```python
from build123d import *

# Parameters (mm, degrees)
SKETCH1_W                      = 560
SKETCH1_H                      = 450
BOSS_EXTRUDE1_DEPTH            = 20
SKETCH3_W                      = 20
SKETCH3_H                      = 450
BOSS_EXTRUDE2_DEPTH            = 120
LPATTERN2_COUNT                = 7
LPATTERN2_PITCH                = 140
LPATTERN5_COUNT                = 2
LPATTERN5_PITCH                = 270
LPATTERN5_COUNT_DIR2           = 14
LPATTERN5_PITCH_DIR2           = 140
SKETCH6_W                      = 450
SKETCH6_H                      = 1000
BOSS_EXTRUDE5_DEPTH            = 20
BOSS_EXTRUDE6_DEPTH            = 450
CUT_EXTRUDE1_REACH             = 1486.158
SKETCH10_R                     = 4.4
CUT_EXTRUDE1_DIRECTION_2_REACH = 1486.158
LPATTERN6_COUNT                = 3
LPATTERN6_PITCH                = 270
SKETCH13_W                     = 315
SKETCH13_H                     = 1.2
CUT_EXTRUDE3_DEPTH             = 20


with BuildPart() as part:
    # Sketch1 → Boss-Extrude1 (new body)
    with BuildSketch(Plane(origin=(0, 0, 0), x_dir=(1, 0, 0), z_dir=(0, 1, 0))):
        Rectangle(SKETCH1_W, SKETCH1_H)
    boss_extrude1 = extrude(amount=BOSS_EXTRUDE1_DEPTH)

    # Sketch3 → Boss-Extrude2 (add)
    with BuildSketch(Plane(origin=(0, 20, 0), x_dir=(1, 0, 0), z_dir=(0, 1, 0))):
        with Locations((-270, 0)):
            Rectangle(SKETCH3_W, SKETCH3_H)
        Rectangle(SKETCH3_W, SKETCH3_H)
        with Locations((270, 0)):
            Rectangle(SKETCH3_W, SKETCH3_H)
    extrude(amount=BOSS_EXTRUDE2_DEPTH)


with BuildPart() as lpattern2_1:
    # LPattern2: pattern copy
    add(part.part.moved(Location(Vector(0, 1, 0) * (1 * LPATTERN2_PITCH))))


with BuildPart() as lpattern2_2:
    # LPattern2: pattern copy
    add(part.part.moved(Location(Vector(0, 1, 0) * (2 * LPATTERN2_PITCH))))


with BuildPart() as lpattern2_3:
    # LPattern2: pattern copy
    add(part.part.moved(Location(Vector(0, 1, 0) * (3 * LPATTERN2_PITCH))))


with BuildPart() as lpattern2_4:
    # LPattern2: pattern copy
    add(part.part.moved(Location(Vector(0, 1, 0) * (4 * LPATTERN2_PITCH))))


with BuildPart() as lpattern2_5:
    # LPattern2: pattern copy
    add(part.part.moved(Location(Vector(0, 1, 0) * (5 * LPATTERN2_PITCH))))


with BuildPart() as lpattern2_6:
    # LPattern2: pattern copy
    add(part.part.moved(Location(Vector(0, 1, 0) * (6 * LPATTERN2_PITCH))))


with BuildPart() as lpattern5_1:
    # LPattern5: pattern copy
    add(boss_extrude1.moved(Location(Vector(1, 0, 0) * (0 * LPATTERN5_PITCH) + Vector(0, 1, 0) * (1 * LPATTERN5_PITCH_DIR2))))


with BuildPart() as lpattern5_2:
    # LPattern5: pattern copy
    add(boss_extrude1.moved(Location(Vector(1, 0, 0) * (0 * LPATTERN5_PITCH) + Vector(0, 1, 0) * (2 * LPATTERN5_PITCH_DIR2))))


with BuildPart() as lpattern5_3:
    # LPattern5: pattern copy
    add(boss_extrude1.moved(Location(Vector(1, 0, 0) * (0 * LPATTERN5_PITCH) + Vector(0, 1, 0) * (3 * LPATTERN5_PITCH_DIR2))))


with BuildPart() as lpattern5_4:
    # LPattern5: pattern copy
    add(boss_extrude1.moved(Location(Vector(1, 0, 0) * (0 * LPATTERN5_PITCH) + Vector(0, 1, 0) * (4 * LPATTERN5_PITCH_DIR2))))


with BuildPart() as lpattern5_5:
    # LPattern5: pattern copy
    add(boss_extrude1.moved(Location(Vector(1, 0, 0) * (0 * LPATTERN5_PITCH) + Vector(0, 1, 0) * (5 * LPATTERN5_PITCH_DIR2))))


with BuildPart() as lpattern5_6:
    # LPattern5: pattern copy
    add(boss_extrude1.moved(Location(Vector(1, 0, 0) * (0 * LPATTERN5_PITCH) + Vector(0, 1, 0) * (6 * LPATTERN5_PITCH_DIR2))))


with BuildPart() as lpattern5_7:
    # LPattern5: pattern copy
    add(boss_extrude1.moved(Location(Vector(1, 0, 0) * (0 * LPATTERN5_PITCH) + Vector(0, 1, 0) * (7 * LPATTERN5_PITCH_DIR2))))


with BuildPart() as lpattern5_8:
    # LPattern5: pattern copy
    add(boss_extrude1.moved(Location(Vector(1, 0, 0) * (1 * LPATTERN5_PITCH) + Vector(0, 1, 0) * (0 * LPATTERN5_PITCH_DIR2))))


with BuildPart() as lpattern5_9:
    # LPattern5: pattern copy
    add(boss_extrude1.moved(Location(Vector(1, 0, 0) * (1 * LPATTERN5_PITCH) + Vector(0, 1, 0) * (1 * LPATTERN5_PITCH_DIR2))))


with BuildPart() as lpattern5_10:
    # LPattern5: pattern copy
    add(boss_extrude1.moved(Location(Vector(1, 0, 0) * (1 * LPATTERN5_PITCH) + Vector(0, 1, 0) * (2 * LPATTERN5_PITCH_DIR2))))


with BuildPart() as lpattern5_11:
    # LPattern5: pattern copy
    add(boss_extrude1.moved(Location(Vector(1, 0, 0) * (1 * LPATTERN5_PITCH) + Vector(0, 1, 0) * (3 * LPATTERN5_PITCH_DIR2))))


with BuildPart() as lpattern5_12:
    # LPattern5: pattern copy
    add(boss_extrude1.moved(Location(Vector(1, 0, 0) * (1 * LPATTERN5_PITCH) + Vector(0, 1, 0) * (4 * LPATTERN5_PITCH_DIR2))))


with BuildPart() as lpattern5_13:
    # LPattern5: pattern copy
    add(boss_extrude1.moved(Location(Vector(1, 0, 0) * (1 * LPATTERN5_PITCH) + Vector(0, 1, 0) * (5 * LPATTERN5_PITCH_DIR2))))


with BuildPart() as lpattern5_14:
    # LPattern5: pattern copy
    add(boss_extrude1.moved(Location(Vector(1, 0, 0) * (1 * LPATTERN5_PITCH) + Vector(0, 1, 0) * (6 * LPATTERN5_PITCH_DIR2))))


with BuildPart() as lpattern5_15:
    # LPattern5: pattern copy
    add(boss_extrude1.moved(Location(Vector(1, 0, 0) * (1 * LPATTERN5_PITCH) + Vector(0, 1, 0) * (7 * LPATTERN5_PITCH_DIR2))))


with BuildPart() as part_1:
    add(part.part)

    # LPattern5 united with what the copies to: union LPattern2_1, LPattern2_2, LPattern2_3, LPattern2_4, LPattern2_5, LPattern2_6, LPattern5_1, LPattern5_2, LPattern5_3, LPattern5_4, LPattern5_5, LPattern5_6, LPattern5_7, LPattern5_8, LPattern5_9, LPattern5_10, LPattern5_11, LPattern5_12, LPattern5_13, LPattern5_14, LPattern5_15
    add(lpattern2_1.part)
    add(lpattern2_2.part)
    add(lpattern2_3.part)
    add(lpattern2_4.part)
    add(lpattern2_5.part)
    add(lpattern2_6.part)
    add(lpattern5_1.part)
    add(lpattern5_2.part)
    add(lpattern5_3.part)
    add(lpattern5_4.part)
    add(lpattern5_5.part)
    add(lpattern5_6.part)
    add(lpattern5_7.part)
    add(lpattern5_8.part)
    add(lpattern5_9.part)
    add(lpattern5_10.part)
    add(lpattern5_11.part)
    add(lpattern5_12.part)
    add(lpattern5_13.part)
    add(lpattern5_14.part)
    add(lpattern5_15.part)

    # Sketch6 → Boss-Extrude5 (add)
    with BuildSketch(Plane(origin=(550, 0, 0), x_dir=(0, 0, -1), z_dir=(1, 0, 0))):
        with Locations((0, 500)):
            Rectangle(SKETCH6_W, SKETCH6_H)
    extrude(amount=-BOSS_EXTRUDE5_DEPTH)

    # Sketch9 → Boss-Extrude6 (add)
    with BuildSketch(Plane.XY.offset(225)):
        Polygon((-260, -482.101596541), (-260, 0), (-280, 0), (-280, -500), (550, -500), (550, 0), (530, 0), (530, -482.101596541), align=None)
    extrude(amount=-BOSS_EXTRUDE6_DEPTH)

    # Cut-Extrude1: up to this face of the body (flat: up to its plane)
    cut_extrude1_end = Plane(part_1.part.faces().sort_by_distance((135, 1000, 0))[0])
    # Sketch10 → Cut-Extrude1 (cut, up to the picked face)
    with BuildSketch(Plane(origin=(0, 860, 0), x_dir=(1, 0, 0), z_dir=(0, 1, 0)), mode=Mode.PRIVATE) as cut_extrude1_sk1:
        with Locations(Location((-250, -215, 0), (0, 0, 270))):
            Circle(SKETCH10_R)
    cut_extrude1_tool1 = split(extrude(cut_extrude1_sk1.sketch, amount=CUT_EXTRUDE1_REACH, mode=Mode.PRIVATE), bisect_by=cut_extrude1_end, keep=Keep.BOTH, mode=Mode.PRIVATE)
    cut_extrude1 = cut_extrude1_tool1.solids().sort_by(Axis((-250, 860, 215), (0, 1, 0)))[0]
    add(cut_extrude1, mode=Mode.SUBTRACT)

    # Cut-Extrude1 direction 2: up to this face of the body (flat: up to its plane)
    cut_extrude1_direction_2_end = Plane(part_1.part.faces().sort_by_distance((135, 0, 0))[0])
    # Sketch10 → Cut-Extrude1 direction 2 (cut, up to the picked face)
    with BuildSketch(Plane(origin=(0, 860, 0), x_dir=(1, 0, 0), z_dir=(0, 1, 0)), mode=Mode.PRIVATE) as cut_extrude1_direction_2_sk1:
        with Locations(Location((-250, -215, 0), (0, 0, 270))):
            Circle(SKETCH10_R)
    cut_extrude1_direction_2_tool1 = split(extrude(cut_extrude1_direction_2_sk1.sketch, amount=-CUT_EXTRUDE1_DIRECTION_2_REACH, mode=Mode.PRIVATE), bisect_by=cut_extrude1_direction_2_end, keep=Keep.BOTH, mode=Mode.PRIVATE)
    cut_extrude1_direction_2 = cut_extrude1_direction_2_tool1.solids().sort_by(Axis((-250, 860, 215), (0, -1, 0)))[0]
    add(cut_extrude1_direction_2, mode=Mode.SUBTRACT)

    # LPattern6: Cut-Extrude1, Cut-Extrude1 direction 2 ×3
    with Locations(*[(i * LPATTERN6_PITCH, 0, 0) for i in range(1, LPATTERN6_COUNT)]):
        add(cut_extrude1, mode=Mode.SUBTRACT)
        add(cut_extrude1_direction_2, mode=Mode.SUBTRACT)

    # Sketch13 → Cut-Extrude3 (cut)
    with BuildSketch(Plane.ZY.offset(280)):
        with Locations((0, -439.4)):
            Rectangle(SKETCH13_W, SKETCH13_H)
    extrude(amount=-CUT_EXTRUDE3_DEPTH, mode=Mode.SUBTRACT)


solid = part_1.part
```
The model under review builds one solid part; all positions refer to its coordinate system, in mm. Round coordinates to 2 decimals unless told otherwise and drop trailing zeros. Write each loop counter-clockwise with the first axis right and the second up, starting at its lowest first coordinate (ties: lowest second). Pieces come first, ordered by that corner, then holes.
(1) We need section B-B on y = -46. Give the boundary of the cut face in (x, z).
(2) We need section C-C on x = 131. Give the number of separate pieces and of enclosed holes in the cut face, and give its area (3 significant figures).
(3) We need section A-A on y = 245.5. Give the boundary of the cut face in (x, z), and give its area (3 significant figures).
(4) Insertion check: pin 1 (7 mm diameter, centred on x = -250, z = 215, fed in from +Y). The pin has a flat end and moves straight along its axis. Give the tip position at first contact, or say it passes through.
(5) Mouldability with a two-part tool opening along Y and no side actions: class faces 1 (the flat face through (403, 420, -3)), 2 (the flat face through (102, 142, 225)), 3 (the flat face through (129, -500, 3)) as +Y half, -Y half, draft (parallel to the pull), parting line (faces both ways), or undercut.
(6) Wall thickness on L1, parallel to X at y = 601.5, z = 142; L2, parallel to X at y = 435.5, z = 215; L3, parallel to X at y = -404, z = 4.5: over which ranges is each line inside the solid? List them lowest first.
Findings below:
1. outline: (-280, -225) - (-260, -225) - (-260, 225) - (-280, 225) - close; (530, -225) - (550, -225) - (550, 225) - (530, 225) - close
2. separate pieces: 9
2. enclosed holes: 0
2. area: 80,100 mm2
3. outline: (-280, -225) - (-260, -225) - (-260, 225) - (-280, 225) - close; (-10, -225) - (10, -225) - (10, 225) - (-10, 225) - close; (260, -225) - (280, -225) - (280, 225) - (260, 225) - close; (530, -225) - (550, -225) - (550, 225) - (530, 225) - close
3. area: 36,000 mm2
4. pin 1: stops at y = -482.1
5. face 1: undercut
5. face 2: draft
5. face 3: -Y half
6. L1: x = -280 to -260, -10 to 10, 260 to 280, 530 to 550
6. L2: x = -280 to -254.4, -245.6 to 15.6, 24.4 to 285.6, 294.4 to 550
6. L3: x = -280 to -260, 530 to 550
